from build123d import *

# Parameters (mm, degrees)
ESQUISSE1_R        = 4.8895
ESQUISSE1_R_2      = 2.032
BOSS_EXTRU_1_DEPTH = 19.71


with BuildPart() as part:
    # Esquisse1 → Boss.-Extru.1 (new, symmetric)
    with BuildSketch(Plane.XY):
        Circle(ESQUISSE1_R)
        Circle(ESQUISSE1_R_2, mode=Mode.SUBTRACT)
    extrude(amount=BOSS_EXTRU_1_DEPTH, both=True)

    # Esquisse2 → Révolution1 (revolve)
    with BuildSketch(Plane(origin=(0, 0, 0), x_dir=(0, 0, -1), z_dir=(1, 0, 0)), mode=Mode.PRIVATE) as r_volution1_sk:
        Polygon((-13.36, 4.8895), (-19.71, 8.0645), (-19.71, 4.8895), align=None)
        Polygon((0, 6.1595), (-6.35, 4.8895), (0, 4.8895), (6.35, 4.8895), align=None)
        Polygon((19.71, 4.8895), (19.71, 8.0645), (13.36, 4.8895), align=None)
    revolve(r_volution1_sk.sketch.rotate(Axis((0, 0, 0), (0, 0, 1)), 90), axis=Axis((0, 0, 0), (0, 0, 1)))


solid = part.part
Geometry: final body of the model. Coordinates: model frame, mm. A direction names the side the tool comes from. Give positions to 0.01 mm unless a question says otherwise; leave off trailing zeros. Write each loop counter-clockwise with the first axis right and the second up, starting at its lowest first coordinate (ties: lowest second). Pieces come first, ordered by that corner, then holes. Notation, with made-up numbers: M -36,74.5 L -3,74.5 A22 ccw -3,107.5 Z; hole C 76,-38.5 d2. An arc over 180 degrees is marked long. Answer in a Markdown table with one row per item. Add a question column.
(1) Section D-D on z = -16.5. Return loops of the section in (x, y).
(2) Reachability of faces 1 (the conical face through (-4.992, -1.572, 4.631)), 2 (the flat face through (-2, 2, 19.71)) from +Z, -Z, +X, -X, +Y, -Y: full face, straight path, thin tool, end or side. Return the list, or none.
(3) Ray query, line 1 (Y direction, x = 0, z = 11); line 2 (X direction, y = -1.5, z = -13); line 3 (Z direction, x = -6.75, y = 3.5). Return the intervals inside material, ascending.
(4) First-contact query: pin 1 (1 mm diameter, centred on x = 0.5, y = 1, fed in from -Z). Flat tip, straight axial feed; report the tip coordinate or a pass-through.
(5) Section A-A on x = 0. Return loops of the section in (y, z), and give its area (3 significant figures).
(6) Section C-C on z = -8. Return loops of the section in (x, y).
(7) Mould query, pull axis Z, two halves, no side actions, for faces 3 (the flat face through (2, -2, -19.71)), 4 (the cylindrical face through (-1.06, -4.773, 9.904)), 5 (the cylindrical face through (-0.44, -1.984, -0.276)). Classes: +Z half, -Z half, draft (parallel to the pull), parting line (faces both ways), or undercut.
Result set:
| question | item | result |
|---|---|---|
| 1 | outline | C 0,0 d12.92; hole C 0,0 d4.06 |
| 2 | face 1 | none |
| 2 | face 2 | +Z, +X, -X, +Y, -Y |
| 3 | line 1 | y = -4.89 to -2.03, 2.03 to 4.89 |
| 3 | line 2 | x = -4.65 to -1.37, 1.37 to 4.65 |
| 3 | line 3 | z = -19.71 to -18.79, 18.79 to 19.71 |
| 4 | pin 1 | passes through |
| 5 | outline | M -8.06,-19.71 L -2.03,-19.71 L -2.03,19.71 L -8.06,19.71 L -4.89,13.36 L -4.89,6.35 L -6.16,0 L -4.89,-6.35 L -4.89,-13.36 Z; M 2.03,-19.71 L 8.06,-19.71 L 4.89,-13.36 L 4.89,-6.35 L 6.16,0 L 4.89,6.35 L 4.89,13.36 L 8.06,19.71 L 2.03,19.71 Z |
| 5 | area | 282 mm^2 |
| 6 | outline | C 0,0 d9.78; hole C 0,0 d4.06 |
| 7 | face 3 | -Z half |
| 7 | face 4 | undercut |
| 7 | face 5 | draft |
